The listing builds one solid part. Answer for the finished solid, in the listing's coordinates (mm). Face numbers are marked on the shaded views. Coordinates: 2 decimals unless noted, no trailing zeros. Write each loop counter-clockwise with the first axis right and the second up, starting at its lowest first coordinate (ties: lowest second). Pieces come first, ordered by that corner, then holes.
from build123d import *

# Parameters (mm, degrees)
F0_W     = 20
F0_H     = 20
F1_DEPTH = 15
F2_R     = 2.25
F3_DEPTH = 15.001
F4_W     = 7
F4_H     = 2.5
F5_DEPTH = 12.5


with BuildPart() as f1:
    # F0 (on Top) → F1 (new body)
    with BuildSketch(Plane.XY):
        Rectangle(F0_W, F0_H)
    extrude(amount=F1_DEPTH)

    # F2 (on face) → F3 (cut, through all)
    with BuildSketch(Plane.XY.offset(15)):
        Circle(F2_R)
    extrude(amount=-F3_DEPTH, mode=Mode.SUBTRACT)

    # F4 (on face) → F5 (cut)
    with BuildSketch(Plane(origin=(-10, 0, 0), x_dir=(0, -1, 0), z_dir=(-1, 0, 0))):
        with Locations((0.59865, 4.25)):
            Rectangle(F4_W, F4_H)
        with Locations((0.59865, 10.75)):
            Rectangle(F4_W, F4_H)
    extrude(amount=-F5_DEPTH, mode=Mode.SUBTRACT)


solid = f1.part
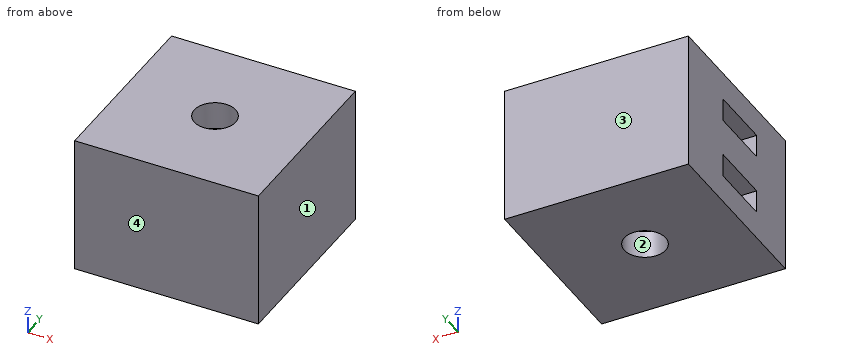
1. Find the intervals of material crossed by L1, parallel to Z at x = -5.75, y = 1; L2, parallel to Y at x = 0, z = 12.95; L3, parallel to Y at x = -5.25, z = 5.25, in increasing order.
Results found:
L1: z = 0 to 3, 5.5 to 9.5, 12 to 15
L2: y = -10 to -2.25, 2.25 to 10
L3: y = -10 to -4.1, 2.9 to 10
2. For a pull along Y with two mould halves and no side action, classify the marked faces 1, 2, 3 and 4 as pulls with the +Y half, pulls with the -Y half, needs draft (parallel to the pull), parting line crosses it, or undercut.
Results found:
face 1: needs draft
face 2: undercut
face 3: pulls with the +Y half
face 4: pulls with the -Y half
3. Section D-D on z = 5 is taken. Give the vertices of the cut face in (x, y), then the cut area to 4 significant figures.
Results found:
outline: (-10, -10) - (10, -10) - (10, 10) - (-10, 10) - (-10, 2.9) - (2.5, 2.9) - (2.5, -4.1) - (-10, -4.1) - close
area: 312.5 mm2
4. Section A-A on x = 0 is taken. Give the vertices of the cut face in (y, z).
Results found:
outline: (-10, 0) - (-2.25, 0) - (-2.25, 3) - (-4.1, 3) - (-4.1, 5.5) - (-2.25, 5.5) - (-2.25, 9.5) - (-4.1, 9.5) - (-4.1, 12) - (-2.25, 12) - (-2.25, 15) - (-10, 15) - close; (2.25, 0) - (10, 0) - (10, 15) - (2.25, 15) - (2.25, 12) - (2.9, 12) - (2.9, 9.5) - (2.25, 9.5) - (2.25, 5.5) - (2.9, 5.5) - (2.9, 3) - (2.25, 3) - close
5. Section C-C on z = 12.75 is taken. Give the vertices of the cut face in (x, y).
Results found:
outline: (-10, -10) - (10, -10) - (10, 10) - (-10, 10) - close; hole circle Ø4.5 at (0, 0)
6. Section B-B on y = 0 is taken. Give the vertices of the cut face in (x, z).
Results found:
outline: (-10, 0) - (-2.25, 0) - (-2.25, 3) - (-10, 3) - close; (-10, 5.5) - (-2.25, 5.5) - (-2.25, 9.5) - (-10, 9.5) - close; (-10, 12) - (-2.25, 12) - (-2.25, 15) - (-10, 15) - close; (2.25, 0) - (10, 0) - (10, 15) - (2.25, 15) - (2.25, 12) - (2.5, 12) - (2.5, 9.5) - (2.25, 9.5) - (2.25, 5.5) - (2.5, 5.5) - (2.5, 3) - (2.25, 3) - close
7. Flat-ended cylindrical pins translate along their axes: P1, Ø1.2, axis at y = 0.5, z = 11, coming from the -X side; P2, Ø3.5, axis at x = 0, y = 0, coming from the +Z side. Find the tip coordinate at first contact, or state that the pin passes through.
Results found:
P1: stops at x = 2.5
P2: passes through
